Part model, mm, in its own coordinate system. A direction names the side the tool comes from. Give positions to 0.01 mm unless a question says otherwise; leave off trailing zeros.
```python
from build123d import *

# Parameters (mm, degrees)
SKETCH4_R                = 11
CUT_EXTRUDE4_DEPTH       = 25.248711
CUT_EXTRUDE5_DEPTH       = 22.610183
BOSS_EXTRUDE1_REACH      = 23.61
BOSS_EXTRUDE1_END_RADIUS = 14
SKETCH5_R                = 1
SKETCH7_W                = 20.713315
SKETCH7_H                = 3.375348
CUT_EXTRUDE6_DEPTH       = 25.228083
CUT_EXTRUDE6_DEPTH_BACK  = 25.228083


with BuildPart() as part:
    # Sketch1 → Revolve1 (revolve)
    with BuildSketch(Plane.XY):
        with BuildLine():
            Line((0, 14), (0, 0))
            Line((0, 0), (14, 0))
            ThreePointArc((14, 0), (9.899495, 9.899495), (0, 14))
        make_face()
    revolve(axis=Axis((0, -754.629412, 0), (0, 1, 0)))

    # Sketch4 → Cut-Extrude4 (cut, through all)
    with BuildSketch(Plane(origin=(0, 0, 0), x_dir=(1, 0, 0), z_dir=(0, 1, 0))):
        with Locations(Location((0, 0, 0), (0, 0, 90))):
            Circle(SKETCH4_R)
    extrude(amount=CUT_EXTRUDE4_DEPTH, mode=Mode.SUBTRACT)

    # Sketch6 → Cut-Extrude5 (cut, through all)
    with BuildSketch(Plane(origin=(0, 0, 0), x_dir=(1, 0, 0), z_dir=(0, 1, 0))):
        with BuildLine():
            Line((-6.517247, 9.056408), (6.517247, 9.056408))
            Line((6.517247, 9.056408), (4, 13.416408))
            ThreePointArc((4, 13.416408), (0, 14), (-4, 13.416408))
            Line((-4, 13.416408), (-6.517247, 9.056408))
        make_face()
    extrude(amount=CUT_EXTRUDE5_DEPTH, mode=Mode.SUBTRACT)

    # Boss-Extrude1: up to this sphere (the profile starts inside it)
    boss_extrude1_end = Location((0, 0, 0)) * Sphere(BOSS_EXTRUDE1_END_RADIUS, mode=Mode.PRIVATE)
    # Sketch5 → Boss-Extrude1 (add, up to the surface)
    with BuildSketch(Plane(origin=(0, 0, 0), x_dir=(1, 0, 0), z_dir=(0, 1, 0)), mode=Mode.PRIVATE) as boss_extrude1_sk1:
        with BuildLine():
            Line((-8.43843, 7.056408), (-1, 7.056408))
            Line((-1, 7.056408), (-1, 1.732051))
            ThreePointArc((-1, 1.732051), (-1.732051, 1), (-2, 0))
            Line((-2, 0), (-12.593387, -6.116095))
            Line((-12.593387, -6.116095), (-11.593387, -7.848145))
            Line((-11.593387, -7.848145), (-1, -1.732051))
            ThreePointArc((-1, -1.732051), (0, -2), (1, -1.732051))
            Line((1, -1.732051), (11.593387, -7.848145))
            Line((11.593387, -7.848145), (12.593387, -6.116095))
            Line((12.593387, -6.116095), (2, 0))
            ThreePointArc((2, 0), (1.732051, 1), (1, 1.732051))
            Line((1, 1.732051), (1, 7.056408))
            Line((1, 7.056408), (8.43843, 7.056408))
            Line((8.43843, 7.056408), (8.43843, 9.056408))
            Line((8.43843, 9.056408), (-8.43843, 9.056408))
            Line((-8.43843, 9.056408), (-8.43843, 7.056408))
        make_face()
        with Locations(Location((0, 0, 0), (0, 0, 90))):
            Circle(SKETCH5_R, mode=Mode.SUBTRACT)
    boss_extrude1_tool1 = extrude(boss_extrude1_sk1.sketch, amount=BOSS_EXTRUDE1_REACH, mode=Mode.PRIVATE) & boss_extrude1_end
    add(boss_extrude1_tool1.solids().sort_by_distance((0, 0, -1.246464))[0])

    # Sketch7 → Cut-Extrude6 (cut, two sides)
    with BuildSketch(Plane.XY) as cut_extrude6_sk:
        with Locations((0.377369, 13.687674)):
            Rectangle(SKETCH7_W, SKETCH7_H)
    extrude(amount=CUT_EXTRUDE6_DEPTH, mode=Mode.SUBTRACT)
    extrude(cut_extrude6_sk.sketch, amount=-CUT_EXTRUDE6_DEPTH_BACK, mode=Mode.SUBTRACT)


solid = part.part
```
1) Saw through at A-A, the plane x = 0. Count the separate pieces of the cut face and the enclosed holes in it, then the cut area to 3 significant figures.
Answers follow:
separate pieces: 3
enclosed holes: 0
area: 125 mm2
2) Two-plate mould, pull along X, no slides. Class faces 3 (the face through (0, 0, -3)), 4 (the face through (6.05, 5.92, 2.34)): +X half, -X half, draft (parallel to the pull), parting line (faces both ways), or undercut.
Answers follow:
face 3: draft
face 4: undercut
3) 3-axis set-ups, long thin cutter, end or side, ignore diameter. For faces 1 (the face through (4.938, 5.916, 4.005)), 2 (the face through (-1, 12, 1)): which of +Z, -Z, +X, -X, +Y, -Y reach the whole face in a straight line?
Answers follow:
face 1: +Y, -Y
face 2: +Z, -Z, +X, -X, +Y
4) Pin check, flat tips, straight feed: pin 1 Ø3 at (y, z) = (3, -0.5) entering from +X; pin 2 Ø1.6 at (x, z) = (0, 0) entering from +Y; pin 3 Ø6 at (y, z) = (8.5, -4.5) entering from -X; pin 4 Ø4 at (y, z) = (8, -6.5) entering from +X. Stop position of each tip, or through.
Answers follow:
pin 1: stops at x = 13.91
pin 2: passes through
pin 3: stops at x = -12.34
pin 4: stops at x = 11.27
5) Wall check: L1, parallel to Z at x = 5, y = 4.25; L2, parallel to X at y = 7.25, z = -3; L3, parallel to X at y = 4.5, z = -4.75. Give the ranges that are in metal, low to high.
Answers follow:
L1: z = -12.37 to -11.68, -9.06 to -7.06, 1.73 to 4.04, 9.8 to 12.37
L2: x = -11.59 to -10.58, -1 to 1, 10.58 to 11.59
L3: x = -12.38 to -9.92, -1 to 1, 9.92 to 12.38
